The listing builds one solid part. Answer for the finished solid, in the listing's coordinates (mm). A direction names the side the tool comes from. Give positions to 0.01 mm unless a question says otherwise; leave off trailing zeros. Write each loop counter-clockwise with the first axis right and the second up, starting at its lowest first coordinate (ties: lowest second). Pieces come first, ordered by that corner, then holes. Notation, with made-up numbers: (51, 15.5) - (74, 15.5) arc R18 ccw to (74, 47.5) - close; hole circle Ø6 at (59.5, 81.25). An arc over 180 degrees is marked (long way). Answer in a Markdown table with one row per item. Add a question column.
from build123d import *

# Parameters (mm, degrees)
SKETCH_W     = 200
SKETCH_H     = 130
SKETCH_R     = 35
SKETCH_R_2   = 1.5
PAD_DEPTH    = 10
SKETCH001_R  = 40
POCKET_DEPTH = 5.5
FILLET_R     = 3


with BuildPart() as part:
    # Sketch → Pad (new body)
    with BuildSketch(Plane.XY):
        with Locations((100, 65)):
            Rectangle(SKETCH_W, SKETCH_H)
        with Locations((100, 65)):
            Circle(SKETCH_R, mode=Mode.SUBTRACT)
        with Locations((45, 115)):
            Circle(SKETCH_R_2, mode=Mode.SUBTRACT)
        with Locations((45, 15)):
            Circle(SKETCH_R_2, mode=Mode.SUBTRACT)
        with Locations((155, 115)):
            Circle(SKETCH_R_2, mode=Mode.SUBTRACT)
        with Locations((155, 15)):
            Circle(SKETCH_R_2, mode=Mode.SUBTRACT)
        with Locations((185, 30)):
            Circle(SKETCH_R_2, mode=Mode.SUBTRACT)
        with Locations((135.353085, 100.338453)):
            Circle(SKETCH_R_2, mode=Mode.SUBTRACT)
        with Locations((64.627773, 29.642413)):
            Circle(SKETCH_R_2, mode=Mode.SUBTRACT)
        with Locations((64.64463, 100.35537)):
            Circle(SKETCH_R_2, mode=Mode.SUBTRACT)
        with Locations((135.352442, 29.63292)):
            Circle(SKETCH_R_2, mode=Mode.SUBTRACT)
        with Locations((175, 20)):
            Circle(SKETCH_R_2, mode=Mode.SUBTRACT)
        with Locations((175, 40)):
            Circle(SKETCH_R_2, mode=Mode.SUBTRACT)
        with Locations((185, 50)):
            Circle(SKETCH_R_2, mode=Mode.SUBTRACT)
        with Locations((175, 90)):
            Circle(SKETCH_R_2, mode=Mode.SUBTRACT)
        with Locations((175, 110)):
            Circle(SKETCH_R_2, mode=Mode.SUBTRACT)
        with Locations((185, 80)):
            Circle(SKETCH_R_2, mode=Mode.SUBTRACT)
        with Locations((185, 100)):
            Circle(SKETCH_R_2, mode=Mode.SUBTRACT)
        with Locations((15, 30)):
            Circle(SKETCH_R_2, mode=Mode.SUBTRACT)
        with Locations((25, 20)):
            Circle(SKETCH_R_2, mode=Mode.SUBTRACT)
        with Locations((25, 40)):
            Circle(SKETCH_R_2, mode=Mode.SUBTRACT)
        with Locations((15, 50)):
            Circle(SKETCH_R_2, mode=Mode.SUBTRACT)
        with Locations((25, 90)):
            Circle(SKETCH_R_2, mode=Mode.SUBTRACT)
        with Locations((25, 110)):
            Circle(SKETCH_R_2, mode=Mode.SUBTRACT)
        with Locations((15, 80)):
            Circle(SKETCH_R_2, mode=Mode.SUBTRACT)
        with Locations((15, 100)):
            Circle(SKETCH_R_2, mode=Mode.SUBTRACT)
    extrude(amount=PAD_DEPTH)

    # Sketch001 (on Face31 of Pad) → Pocket (cut)
    with BuildSketch(Plane.XY.offset(10)):
        with Locations((100, 65)):
            Circle(SKETCH001_R)
    extrude(amount=-POCKET_DEPTH, mode=Mode.SUBTRACT)

    # Fillet
    fillet_edges = [part.edges().sort_by_distance(p)[0] for p in [
        (200, 0, 5),
        (200, 130, 5),
        (0, 0, 5),
        (0, 130, 5),
    ]]
    fillet(fillet_edges, radius=FILLET_R)


solid = part.part
1. A tool of negligible diameter and unlimited length cuts with its end or side. For faces 5 (the face through (99, 109, 10)), 6 (the face through (99.8, 29.6, 4.5)), from which of +Z, -Z, +X, -X, +Y, -Y can it reach the whole face along a straight path? Write none if from no direction.
2. Straight lines are drawn through the part: L1, parallel to Y at x = 175, z = 2.5; L2, parallel to X at y = 115, z = 3.25; L3, parallel to Y at x = 185, z = 3. For each, find the intervals that lie inside material, in ascending order. Write a range as [from, to].
3. Section C-C (z = 8) is taken. State how many separate pieces and enclosed holes the cut face has, and give its area (3 significant figures).
4. The mould has two halves that part along X. Classify faces 1 (the face through (118.82, 94.51, 2.22)), 2 (the face through (138.153, 77.015, 7.288)), 3 (the face through (99, 130, 5)), 4 (the face through (0, 64, 5)): +X half, -X half, draft (parallel to the pull), parting line (faces both ways), or undercut.
5. Section A-A (x = 100) is taken. Give the vertices of the cut face in (y, z).
6. Section B-B (y = 85) is taken. Give the vertices of the cut face in (x, z).
7. Given pin 1 Ø5 at (x, y) = (155, 115) entering from -Z; pin 2 Ø2.5 at (x, y) = (175, 20) entering from +Z, each flat-ended and moving along its own axis, determine where each tip first touches the part or whether it passes through.
Geometry check:
| question | item | result |
|---|---|---|
| 1 | face 5 | +Z, +X, -X, +Y, -Y |
| 1 | face 6 | +Z |
| 2 | L1 | [0, 18.5], [21.5, 38.5], [41.5, 88.5], [91.5, 108.5], [111.5, 130] |
| 2 | L2 | [0, 43.5], [46.5, 153.5], [156.5, 200] |
| 2 | L3 | [0, 28.5], [31.5, 48.5], [51.5, 78.5], [81.5, 98.5], [101.5, 130] |
| 3 | separate pieces | 1 |
| 3 | enclosed holes | 25 |
| 3 | area | 20,800 mm² |
| 4 | face 1 | undercut |
| 4 | face 2 | undercut |
| 4 | face 3 | draft |
| 4 | face 4 | -X half |
| 5 | outline | (0, 0) - (30, 0) - (30, 4.5) - (25, 4.5) - (25, 10) - (0, 10) - close; (100, 0) - (130, 0) - (130, 10) - (105, 10) - (105, 4.5) - (100, 4.5) - close |
| 6 | outline | (0, 0) - (71.28, 0) - (71.28, 4.5) - (65.36, 4.5) - (65.36, 10) - (0, 10) - close; (128.72, 0) - (200, 0) - (200, 10) - (134.64, 10) - (134.64, 4.5) - (128.72, 4.5) - close |
| 7 | pin 1 | z = 0 |
| 7 | pin 2 | through |
